Verification items for the finished model (mm, model axes). Coordinates: 2 decimals unless noted, no trailing zeros. Write each loop counter-clockwise with the first axis right and the second up, starting at its lowest first coordinate (ties: lowest second). Pieces come first, ordered by that corner, then holes. Notation, with made-up numbers: (-33, 13.25) - (-6, 13.25) arc R18 ccw to (-6, 42.25) - close; hole circle Ø9 at (34.25, 77.25). An arc over 180 degrees is marked (long way). Use CSV: the item, a comma, the result in double quotes. Start each with the question number.
```python
from build123d import *

# Parameters (mm, degrees)
BOSS_EXTRUDE1_DEPTH = 3.175


with BuildPart() as part:
    # Sketch1 → Boss-Extrude1 (new body)
    with BuildSketch(Plane.XY):
        Polygon((0, 0), (6.35, 0), (6.35, -3.03), (31.35, -3.03), (31.35, -9.38), (56.35, -9.38), (56.35, -3.03), (81.35, -3.03), (81.35, -9.38), (106.35, -9.38), (106.35, -3.03), (131.35, -3.03), (131.35, -9.38), (156.35, -9.38), (156.35, -3.03), (181.35, -3.03), (181.35, -9.38), (206.35, -9.38), (206.35, -3.03), (231.35, -3.03), (231.35, -9.38), (256.35, -9.38), (256.35, -3.03), (281.35, -3.03), (281.35, -9.38), (306.35, -9.38), (306.35, -3.03), (331.35, -3.03), (331.35, -9.38), (356.35, -9.38), (356.35, -3.03), (381.35, -3.03), (381.35, -9.38), (406.35, -9.38), (406.35, -3.03), (409.425, -3.028710343), (409.425, 2.97e-07), (415.775, 2.97e-07), (415.775, 5), (409.42, 5), (0, 5), align=None)
    extrude(amount=BOSS_EXTRUDE1_DEPTH)


solid = part.part
```
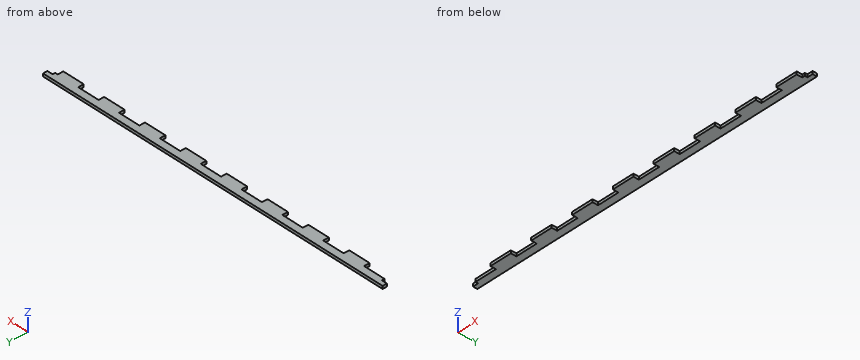
Q1. Gauge pin test, flat ends, axial feed: pin 1 (1.5 mm diameter, centred on y = -3.5, z = 1, fed in from +X) (3 decimals); pin 2 (1 mm diameter, centred on y = -7.5, z = 1.5, fed in from +X); pin 3 (1.6 mm diameter, centred on x = 69.5, z = 1, fed in from -Y). Record the tip position at first contact, or that the pin passes through.
Q2. Cross-section at A-A (y = -5.5). State how many separate pieces and enclosed holes the cut face has, plus the area to 3 significant figures.
Q3. Scan lines: line 1 along Y through (x, z) = (169.5, 1.7); line 2 along X through (y, z) = (-0.5, 0.5) (3 decimals). Record each from-to range of solid material in increasing order. Write a range as from..to.
Q4. Cross-section at B-B (x = 269.5). Record the cut outline in (y, z) (3 decimals), plus the area to 3 significant figures.
Reply:
1,pin 1,"x = 409.425"
1,pin 2,"x = 406.35"
1,pin 3,"y = -3.03"
2,separate pieces,"8"
2,enclosed holes,"0"
2,area,"635 mm^2"
3,line 1,"-3.03..5"
3,line 2,"6.35..409.425"
4,outline,"(-3.03, 0) - (5, 0) - (5, 3.175) - (-3.03, 3.175) - close"
4,area,"25.5 mm^2"
